CAD build for the part. Positions are in the model's coordinates, mm. Coordinates: 2 decimals unless noted, no trailing zeros. Loops run counter-clockwise (first coordinate to the right, second up) from the corner with the lowest first, then second, coordinate; pieces in that order, holes last. Notation, with made-up numbers: (-27, 52) -> (-1, 52) arc R17 ccw to (-1, 59) -> close; hole circle Ø7 at (42.25, 40.25). An arc over 180 degrees is marked (long way). Answer as a JSON object with one key per item and string values. Group by question number.
from build123d import *

# Parameters (mm, degrees)
SKETCH_1_R      = 2
SKETCH_1_R_2    = 6.5
EXTRUDE_1_DEPTH = 2
FILLET_1_R      = 10


with BuildPart() as part:
    # 草图1 → 凸台-拉伸1 (new body)
    with BuildSketch(Plane.XY):
        Polygon((-29.269334238, -5), (44.269334238, -5), (36.813954208, 21), (-21.813954208, 21), align=None)
        with Locations((15, 17)):
            Circle(SKETCH_1_R, mode=Mode.SUBTRACT)
        with Locations((15, 0)):
            Circle(SKETCH_1_R, mode=Mode.SUBTRACT)
        Circle(SKETCH_1_R, mode=Mode.SUBTRACT)
        with Locations((0, 17)):
            Circle(SKETCH_1_R, mode=Mode.SUBTRACT)
        with Locations((7.5, 8)):
            Circle(SKETCH_1_R_2, mode=Mode.SUBTRACT)
    extrude(amount=EXTRUDE_1_DEPTH)

    # 圆角1
    fillet_1_edges = [part.edges().sort_by_distance(p)[0] for p in [
        (-21.813954208, 21, 1),
        (36.813954208, 21, 1),
    ]]
    fillet(fillet_1_edges, radius=FILLET_1_R)


solid = part.part
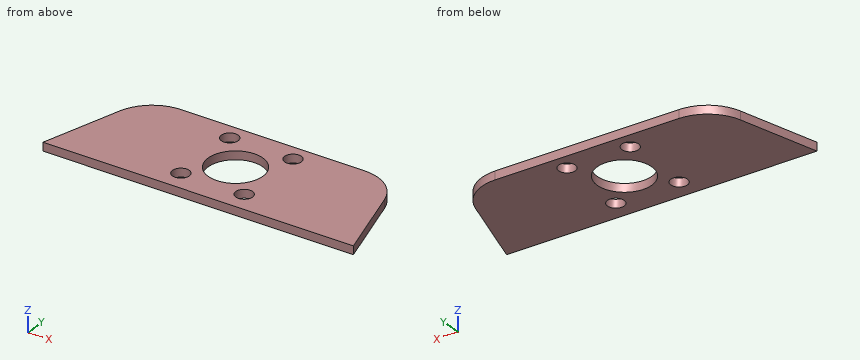
Item 1: Band-saw the part on B-B, the plane x = 0. List the corners of the cut face in (y, z).
Item 2: Drill centre lines: L1, parallel to Y at x = 0, z = 1.5; L2, parallel to X at y = 18, z = 1.3; L3, parallel to X at y = -1.5, z = 1.4. Where is each one in solid material? Low to high.
Item 3: Flat gauge pins, fed straight in: P1, Ø1, axis at x = -16, z = 1, coming from the +Y side; P2, Ø3.5, axis at x = 0, y = 17, coming from the -Z side. Where does each tip first touch, or does it go through?
Item 4: Band-saw the part on D-D, the plane y = 17. List the corners of the cut face in (x, z).
Item 5: Band-saw the part on C-C, the plane z = 1.15. List the corners of the cut face in (x, y), and give its area (3 significant figures).
Item 6: Band-saw the part on A-A, the plane x = 10. List the corners of the cut face in (y, z), and give its area (3 significant figures).
Reply:
{
 "1": {"outline": "(-5, 0) -> (-2, 0) -> (-2, 2) -> (-5, 2) -> close; (2, 0) -> (15, 0) -> (15, 2) -> (2, 2) -> close; (19, 0) -> (21, 0) -> (21, 2) -> (19, 2) -> close"},
 "2": {"L1": "-5 to -2, 2 to 15, 19 to 21", "L2": "-21.42 to -1.73, 1.73 to 13.27, 16.73 to 36.42", "L3": "-28.27 to -1.32, 1.32 to 13.68, 16.32 to 43.27"},
 "3": {"P1": "y = 20.93", "P2": "through"},
 "4": {"outline": "(-22.28, 0) -> (-2, 0) -> (-2, 2) -> (-22.28, 2) -> close; (2, 0) -> (13, 0) -> (13, 2) -> (2, 2) -> close; (17, 0) -> (37.28, 0) -> (37.28, 2) -> (17, 2) -> close"},
 "5": {"outline": "(-29.27, -5) -> (44.27, -5) -> (38.89, 13.76) arc R10 ccw to (29.28, 21) -> (-14.28, 21) arc R10 ccw to (-23.89, 13.76) -> close; hole circle Ø4 at (0, 0); hole circle Ø4 at (0, 17); hole circle Ø13 at (7.5, 8); hole circle Ø4 at (15, 0); hole circle Ø4 at (15, 17)", "area": "1,510 mm²"},
 "6": {"outline": "(-5, 0) -> (2, 0) -> (2, 2) -> (-5, 2) -> close; (14, 0) -> (21, 0) -> (21, 2) -> (14, 2) -> close", "area": "28.0 mm²"}
}
